Input: dimensioned drawing with shaded views. Units: mm. Origin: part minimum x, y, z. Give positions to 0.01 mm unless a question says otherwise; leave off trailing zeros. Write each loop counter-clockwise with the first axis right and the second up, starting at its lowest first coordinate (ties: lowest second). Pieces come first, ordered by that corner, then holes. Notation, with made-up numbers: (37.5, 71.25) -> (82.5, 71.25) arc R31 ccw to (82.5, 98.25) -> close; hole circle Ø10 at (-13, 75). An arc over 180 degrees is marked (long way). Answer as a JSON object with one key per item and string values.
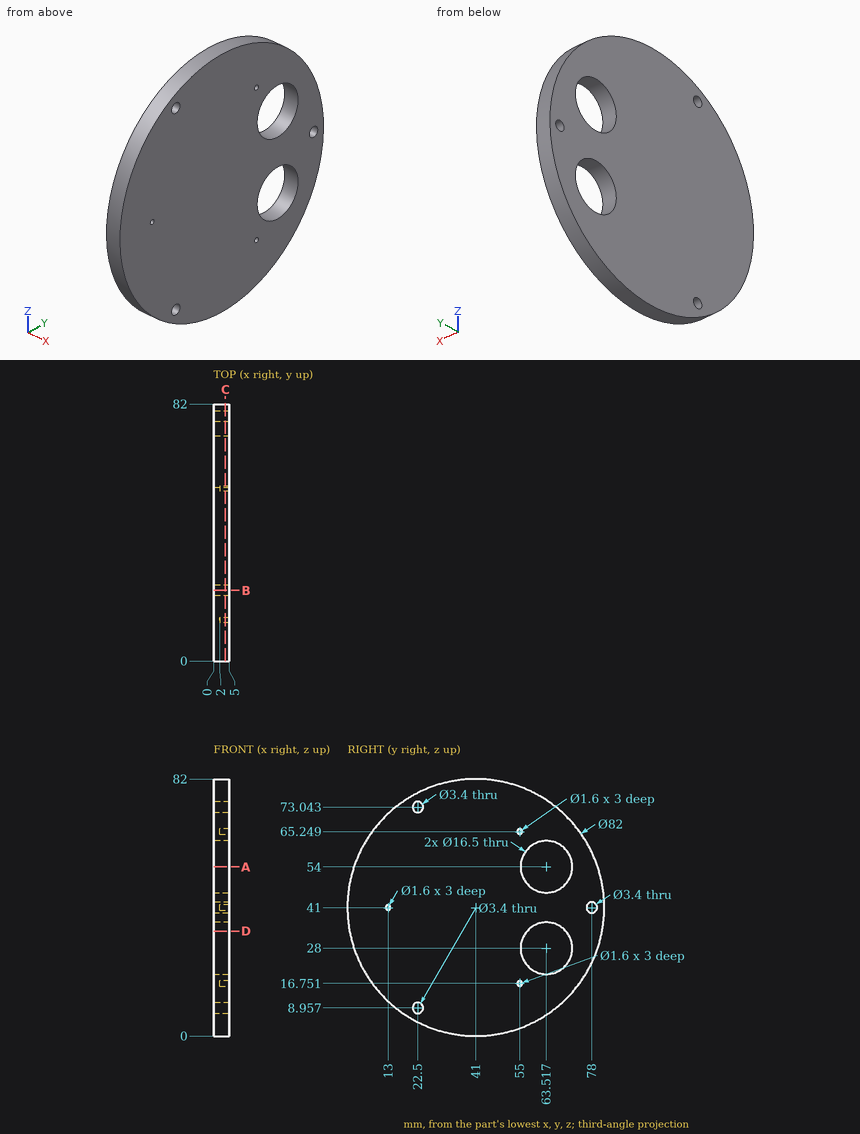
Q1. Cut plane D-D (z = 33.5). Return the cut outline in (x, y).
Values:
{"outline": "(0, 0.69) -> (5, 0.69) -> (5, 57.37) -> (0, 57.37) -> close; (0, 69.67) -> (5, 69.67) -> (5, 81.31) -> (0, 81.31) -> close"}
Q2. First-contact query: P1, Ø1, axis at x = 4.5, y = 45, coming from the -Z side; P2, Ø1.5, axis at x = 1.5, z = 26.5, coming from the -Y side (1 decimal); P3, Ø10, axis at y = 63.52, z = 28, coming from the -X side; P4, Ø2, axis at x = 3, y = 20.5, coming from the +Z side (1 decimal). Flat tips, straight axial feed; report the tip coordinate or a pass-through.
Values:
{"P1": "z = 0.15", "P2": "y = 2.4", "P3": "through", "P4": "z = 77.1"}
Q3. Cut plane A-A (z = 54). Return the cut outline in (x, y) (1 decimal).
Values:
{"outline": "(0, 2.1) -> (5, 2.1) -> (5, 55.3) -> (0, 55.3) -> close; (0, 71.8) -> (5, 71.8) -> (5, 79.9) -> (0, 79.9) -> close"}
Q4. Material intervals for L1, parallel to Y at x = 3.7, z = 41; L2, parallel to Z at x = 3.1, y = 55 (1 decimal); L3, parallel to Z at x = 2.8, y = 56.5 (1 decimal), sorted ascending. Write a range as from..to.
Values:
{"L1": "0..12.2, 13.8..76.3, 79.7..82", "L2": "2.5..16, 17.6..64.4, 66..79.5", "L3": "3..23.7, 32.3..49.7, 58.3..79"}
Q5. Cut plane B-B (y = 22.5). Return the cut outline in (x, z), and give its area (3 significant figures).
Values:
{"outline": "(0, 4.41) -> (5, 4.41) -> (5, 7.26) -> (0, 7.26) -> close; (0, 10.66) -> (5, 10.66) -> (5, 71.34) -> (0, 71.34) -> close; (0, 74.74) -> (5, 74.74) -> (5, 77.59) -> (0, 77.59) -> close", "area": "332 mm²"}
Q6. Cut plane C-C (x = 3.7). State how many separate pieces and enclosed holes the cut face has, and give its area (3 significant figures).
Values:
{"separate pieces": "1", "enclosed holes": "8", "area": "4,820 mm²"}
